```python
from build123d import *

# Parameters (mm, degrees)
FILLET1_R       = 0.6
FILLET2_R       = 0.6
HEX_2_DEPTH     = 6
THDSCHPAT_COUNT = 12
THDSCHPAT_PITCH = 1.645833333


with BuildPart() as part:
    # BodySke → Base-Revolve (revolve)
    with BuildSketch(Plane.XY):
        Polygon((0, 0), (0, 9), (10, 9), (10, 6), (34.036, 6), (35, 5.036), (35, 0), align=None)
    revolve(axis=Axis((-31.75, 0, 0), (1, 0, 0)))

    # Fillet1
    fillet1_edges = [part.edges().sort_by_distance(p)[0] for p in [
        (10, -6, 0),
    ]]
    fillet(fillet1_edges, radius=FILLET1_R)

    # Fillet2
    fillet2_edges = [part.edges().sort_by_distance(p)[0] for p in [
        (0, -9, 0),
    ]]
    fillet(fillet2_edges, radius=FILLET2_R)

    # Sketch2 → Hex-PreBroach (revolve, cut)
    with BuildSketch(Plane.XY):
        Polygon((0, 5.0575), (6, 5.0575), (8.919948986, 0), (0, 0), align=None)
    revolve(axis=Axis((0, 0, 0), (1, 0, 0)), mode=Mode.SUBTRACT)

    # Sketch3 → Hex 2 (cut)
    with BuildSketch(Plane(origin=(0, 0, 0), x_dir=(0, 0.5, 0.866025404), z_dir=(-1, 0, 0))):
        Polygon((2.919948986, 5.0575), (-2.919948986, 5.0575), (-5.839897973, 0), (-2.919948986, -5.0575), (2.919948986, -5.0575), (5.839897973, 0), align=None)
    extrude(amount=-HEX_2_DEPTH, mode=Mode.SUBTRACT)

    # ThdSchSke → ThreadSchematic (revolve, cut)
    with BuildSketch(Plane.XY):
        Polygon((15.25, -5.036), (14.574999933, -6), (14.574999933, -7.5), (15.925000067, -7.5), (15.925000067, -6), align=None)
    threadschematic = revolve(axis=Axis((-3.175, 0, 0), (1, 0, 0)), mode=Mode.SUBTRACT)

    # ThdSchPat: ThreadSchematic ×12
    with Locations(*[(i * THDSCHPAT_PITCH, 0, 0) for i in range(1, THDSCHPAT_COUNT)]):
        add(threadschematic, mode=Mode.SUBTRACT)


solid = part.part
```
CAD build for the part. Positions are in the model's coordinates, mm. Coordinates: 2 decimals unless noted, no trailing zeros. Loops run counter-clockwise (first coordinate to the right, second up) from the corner with the lowest first, then second, coordinate; pieces in that order, holes last. Notation, with made-up numbers: (11, -27.75) - (39, -27.75) arc R23 ccw to (39, 8.25) - close; hole circle Ø1 at (36, 14). An arc over 180 degrees is marked (long way). Use CSV: the item, a comma, the result in double quotes. Start each with the question number.
Q1. Drop flat-ended pins along their axis: P1, Ø6, axis at x = 26.5, z = -6, coming from the +Y side; P2, Ø3, axis at y = 2.5, z = 3.5, coming from the -X side; P3, Ø1, axis at x = 30, y = 0, coming from the +Z side; P4, Ø0.8, axis at y = 1, z = -4, coming from the -X side. Give the stop position or say it passes through.
Q2. Two-plate mould, pull along Y, no slides. Class faces 1 (the flat face through (2.96, -4.36, -2.56)), 2 (the flat face through (0, 4, -4)), 3 (the flat face through (2.96, 4.36, 2.56)), 4 (the cylindrical face through (5.366, -1.172, 8.923)): +Y half, -Y half, draft (parallel to the pull), parting line (faces both ways), or undercut.
Q3. Cut at B-B, the plane x = 13.5. List the corners of the cut face in (y, z), then the cut area to 3 significant figures.
Q4. Probe probe 1 along Y at (x, z) = (31, -0.25); probe 2 along Z at (x, y) = (17, -1.25); probe 3 along X at (y, z) = (-6.75, -1.5). List the from-to ranges inside material, lowest first. Write a range as from..to.
Q5. Cut at A-A, the plane x = 6.5. List the corners of the cut face in (y, z), then the cut area to 3 significant figures.
Here are the results:
1,P1,"y = 5.18"
1,P2,"x = 0"
1,P3,"z = 5.84"
1,P4,"x = 6.31"
2,face 1,"undercut"
2,face 2,"draft"
2,face 3,"undercut"
2,face 4,"parting line"
3,outline,"circle Ø12 at (0, 0)"
3,area,"113 mm2"
4,probe 1,"-5.99..5.99"
4,probe 2,"-5.03..5.03"
4,probe 3,"0..10"
5,outline,"circle Ø18 at (0, 0); hole circle Ø8.38 at (0, 0)"
5,area,"199 mm2"
